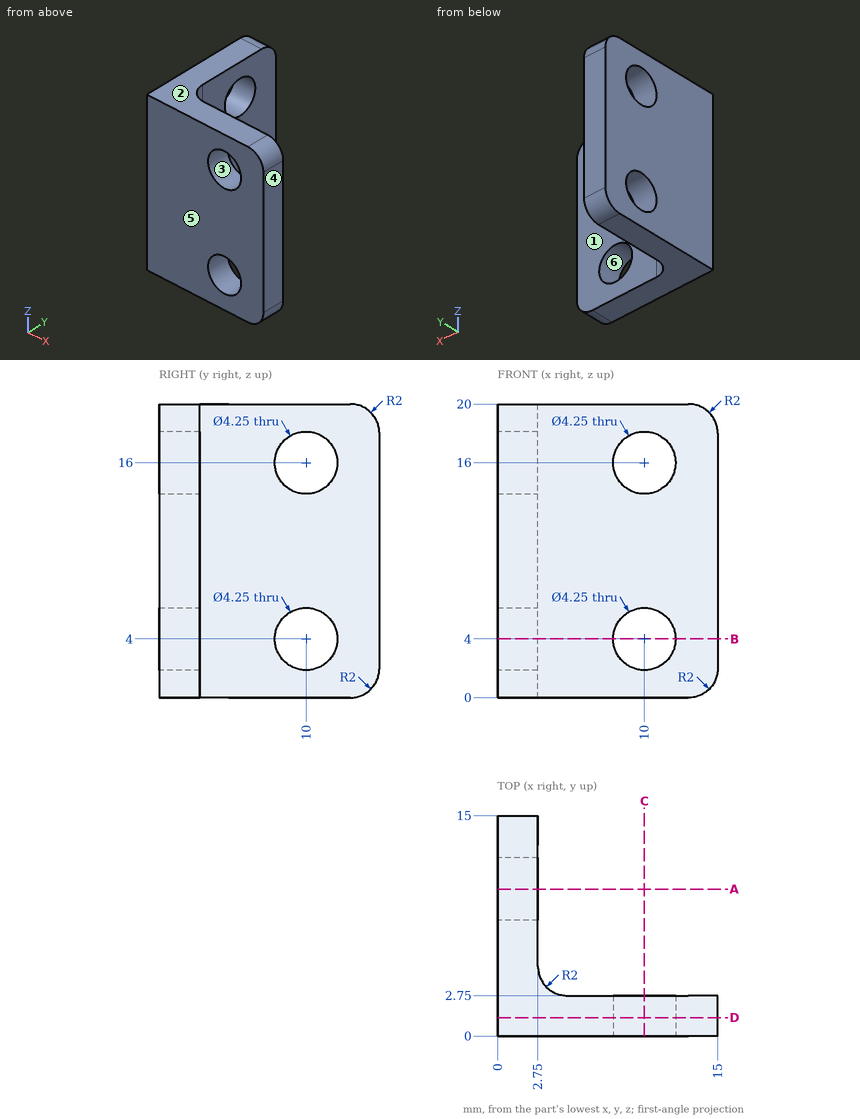
Input: dimensioned drawing with shaded views. Units: mm. Origin: part minimum x, y, z. A direction names the side the tool comes from. Round coordinates to 2 decimals unless told otherwise and drop trailing zeros. Loops run counter-clockwise (first coordinate to the right, second up) from the corner with the lowest first, then second, coordinate; pieces in that order, holes last. Notation, with made-up numbers: M 68,47.25 L 126,47.25 A33 ccw 126,85.25 Z; hole C -11,-11.75 d9. An arc over 180 degrees is marked long. Answer in a Markdown table with one row per item. Add a question column.
1. Mould query, pull axis X, two halves, no side actions, for the marked faces 3, 4, 5 and 6. Classes: released by +X, released by -X, zero draft, split by the parting line, or undercut.
2. Section D-D (y = 1.25). Output: boundary loops of the cut face in (x, z) (3 decimals), and give its area (3 significant figures).
3. Section B-B (z = 4). Output: boundary loops of the cut face in (x, y) (3 decimals), and give its area (3 significant figures).
4. Ray query, probe 1 along Z at (x, y) = (2.5, 11.5); probe 2 along Y at (x, z) = (0.7, 4) (3 decimals); probe 3 along Y at (x, z) = (12.25, 16). Return the intervals inside material, ascending.
5. Contact query for flat-ended pins moving along their axis: pin 1 (3 mm diameter, centred on x = 8, z = 14.5, fed in from +Y); pin 2 (5 mm diameter, centred on y = 10.5, z = 14.5, fed in from +X). Output: stop coordinate, or through.
6. Set-up query: the marked faces 1 and 2. Return all of +Z, -Z, +X, -X, +Y, -Y with unobstructed straight access to the full face (end or side cutting, diameter ignored); none if empty.
7. Section A-A (y = 10). Output: boundary loops of the cut face in (x, z) (3 decimals), and give its area (3 significant figures).
Values follow:
| question | item | result |
|---|---|---|
| 1 | face 3 | undercut |
| 1 | face 4 | released by +X |
| 1 | face 5 | zero draft |
| 1 | face 6 | undercut |
| 2 | outline | M 0,0 L 13,0 A2 ccw 15,2 L 15,18 A2 ccw 13,20 L 0,20 Z; hole C 10,4 d4.25; hole C 10,16 d4.25 |
| 2 | area | 270 mm^2 |
| 3 | outline | M 0,0 L 7.875,0 L 7.875,2.75 L 4.75,2.75 A2 cw 2.75,4.75 L 2.75,7.875 L 0,7.875 Z; M 0,12.125 L 2.75,12.125 L 2.75,15 L 0,15 Z; M 12.125,0 L 15,0 L 15,2.75 L 12.125,2.75 Z |
| 3 | area | 52.4 mm^2 |
| 4 | probe 1 | 0 to 2.49, 5.51 to 14.49, 17.51 to 20 |
| 4 | probe 2 | 0 to 7.875, 12.125 to 15 |
| 4 | probe 3 | 0 to 2.75 |
| 5 | pin 1 | y = 2.75 |
| 5 | pin 2 | x = 2.75 |
| 6 | face 1 | +Z, -Z, +X, +Y |
| 6 | face 2 | +Z, +X, -X, +Y, -Y |
| 7 | outline | M 0,0 L 2.75,0 L 2.75,1.875 L 0,1.875 Z; M 0,6.125 L 2.75,6.125 L 2.75,13.875 L 0,13.875 Z; M 0,18.125 L 2.75,18.125 L 2.75,20 L 0,20 Z |
| 7 | area | 31.6 mm^2 |
